from build123d import *

# Parameters (mm, degrees)
PAD_DEPTH          = 70
SKETCH002_W        = 20
SKETCH002_H        = 20
PAD001_DEPTH       = 2
SKETCH003_R        = 1
POCKET_DEPTH       = 5
POLARPATTERN_COUNT = 4


with BuildPart() as pad:
    # Sketch001 → Pad (new body)
    with BuildSketch(Plane.XY):
        with BuildLine():
            Line((-5, 4), (-5, 5))
            Line((-5, 5), (5, 5))
            Line((5, 5), (5, 4))
            Line((5, 4), (1.6, 4))
            ThreePointArc((1.6, 4), (0.751472, 3.648528), (0.4, 2.8))
            Line((0.4, 2.8), (0.4, -2.8))
            ThreePointArc((0.4, -2.8), (0.751472, -3.648528), (1.6, -4))
            Line((1.6, -4), (5, -4))
            Line((5, -4), (5, -5))
            Line((5, -5), (-5, -5))
            Line((-5, -5), (-5, -4))
            Line((-5, -4), (-1.6, -4))
            ThreePointArc((-1.6, -4), (-0.751472, -3.648528), (-0.4, -2.8))
            Line((-0.4, -2.8), (-0.4, 2.8))
            ThreePointArc((-0.4, 2.8), (-0.751472, 3.648528), (-1.6, 4))
            Line((-1.6, 4), (-5, 4))
        make_face()
    extrude(amount=PAD_DEPTH)


with BuildPart() as fusion:
    # Sketch002 → Pad001 (new body)
    with BuildSketch(Plane.XY):
        Rectangle(SKETCH002_W, SKETCH002_H)
    extrude(amount=PAD001_DEPTH)

    # Sketch003 → Pocket (cut)
    with BuildSketch(Plane.XY.offset(2)):
        with Locations((-7, 7)):
            Circle(SKETCH003_R)
    pocket = extrude(amount=-POCKET_DEPTH, mode=Mode.SUBTRACT)

    # PolarPattern: Pocket ×4 about axis
    polarpattern_axis = Axis((0, 0, 2), (0, 0, 1))
    for i in range(1, POLARPATTERN_COUNT):
        add(pocket.rotate(polarpattern_axis, i * 360 / POLARPATTERN_COUNT), mode=Mode.SUBTRACT)

    # Fusion: union Pad
    add(pad.part)


solid = fusion.part
Build history of the part. All positions in model axes, mm. A direction names the side the tool comes from. Coordinates: 2 decimals unless noted, no trailing zeros. Order: outer loops, then holes, each group sorted by start corner. A loop starts at its lowest first (then second) coordinate and runs counter-clockwise, first axis right, second up. Notation, with made-up numbers: (7, -38) - (15, -38) arc R12 cw to (15, -31) - close; hole circle Ø2 at (-34, -39). An arc over 180 degrees is marked (long way). Put each result on its own line as item: value.
1. Pull direction Y, two halves, no side cores. Call faces 4 (the face through (-8, -7, 1)), 5 (the face through (-0.742, 3.639, 35.524)), 6 (the face through (0, 5, 36)), 7 (the face through (0, -10, 1)): pulls with the +Y half, pulls with the -Y half, needs draft (parallel to the pull), parting line crosses it, or undercut.
Answer sheet:
face 4: undercut
face 5: undercut
face 6: pulls with the +Y half
face 7: pulls with the -Y half
2. Probe line 1 along Y through (x, z) = (-7, 1.1); line 2 along Y through (x, z) = (2, 40). List the from-to ranges inside material, lowest first. Write a range as [from, to].
Answer sheet:
line 1: y = [-10, -8], [-6, 6], [8, 10]
line 2: y = [-5, -4], [4, 5]
3. Drop flat-ended pins along their axis: P1, Ø1.6, axis at x = 7, y = 7, coming from the -Z side; P2, Ø6, axis at x = -4, y = -3.5, coming from the -Z side; P3, Ø1.1, axis at y = 4.5, z = 42.5, coming from the -X side; P4, Ø0.5, axis at y = -4.5, z = 49, coming from the +X side. Give the stop position or say it passes through.
Answer sheet:
P1: passes through
P2: stops at z = 0
P3: stops at x = -5
P4: stops at x = 5
4. Saw through at C-C (z = 58). Write the cut outline in (x, y), and give its area (3 significant figures).
Answer sheet:
outline: (-5, -5) - (5, -5) - (5, -4) - (1.6, -4) arc R1.2 cw to (0.4, -2.8) - (0.4, 2.8) arc R1.2 cw to (1.6, 4) - (5, 4) - (5, 5) - (-5, 5) - (-5, 4) - (-1.6, 4) arc R1.2 cw to (-0.4, 2.8) - (-0.4, -2.8) arc R1.2 cw to (-1.6, -4) - (-5, -4) - close
area: 27.6 mm^2
5. Saw through at A-A (x = 7). Write the cut outline in (y, z), and give its area (3 significant figures).
Answer sheet:
outline: (-10, 0) - (-8, 0) - (-8, 2) - (-10, 2) - close; (-6, 0) - (6, 0) - (6, 2) - (-6, 2) - close; (8, 0) - (10, 0) - (10, 2) - (8, 2) - close
area: 32.0 mm^2
6. Saw through at D-D (y = 1.5). Write the cut outline in (x, z).
Answer sheet:
outline: (-10, 0) - (10, 0) - (10, 2) - (0.4, 2) - (0.4, 70) - (-0.4, 70) - (-0.4, 2) - (-10, 2) - close
7. Tool access for faces 1 (the face through (-0.4, 0, 36)), 2 (the face through (0, 10, 1)), 3 (the face through (0.761, 3.658, 35.524)): list every direction of +Z, -Z, +X, -X, +Y, -Y with a clear straight run to the whole face (end or side of a thin tool).
Answer sheet:
face 1: +Z, -X
face 2: +Z, -Z, +X, -X, +Y
face 3: +Z, +X
